The model under review builds one solid part; all positions refer to its coordinate system, in mm. A direction names the side the tool comes from. Round coordinates to 2 decimals unless told otherwise and drop trailing zeros. Loops run counter-clockwise (first coordinate to the right, second up) from the corner with the lowest first, then second, coordinate; pieces in that order, holes last. Notation, with made-up numbers: M 20.25,80 L 55.25,80 A5 ccw 55.25,84 Z; hole C 47.25,56 d11. An arc over 180 degrees is marked long. Return JSON: item names as keys, results as strings. Group by question number.
Q1. Consider section A-A (x = 10). State the section outline as (y, z) points, and give its area (3 significant figures).
Q2. Clearance check with flat-ended pins moving along their axes: pin 1 Ø4.5 at (x, z) = (10, 7.5) entering from +Y; pin 2 Ø0.8 at (y, z) = (0.5, 5.5) entering from -X; pin 3 Ø3 at (x, z) = (14, 3) entering from +Y. State where each tip first meets the part, or that it passes through.
Q3. Consider section C-C (y = 2.5). State the section outline as (x, z) points.
Q4. Draft analysis for pull direction Z (two halves, no side actions). For faces 1 (the face through (32, 0, 8)), 2 (the face through (32.61, 0.45, 0.43)), 3 (the face through (8, 4, 9)), state which applies: pulls with the +Z half, pulls with the -Z half, needs draft (parallel to the pull), parting line crosses it, or undercut.
Q5. Consider section D-D (z = 10.75). State the section outline as (x, y) points, and give its area (3 significant figures).
Q6. For faces 4 (the face through (25, 7, 8)), 5 (the face through (20, 4, 0)), 6 (the face through (25, 1, 8)), list the 3-axis set-ups (+Z, -Z, +X, -X, +Y, -Y) from which the entire face can be reached by the end or side of a thin tool; tool diameter is ignored.
Q7. To check wall thickness, follow line 1 along X through (y, z) = (5.25, 7.5); line 2 along Y through (x, z) = (14, 11.5); line 3 along X through (y, z) = (4, 6). State the ranges of each line that lie inside material, in increasing order.
Q8. Consider section B-B (z = 7.5). State the section outline as (x, y) points.
from build123d import *

# Parameters (mm, degrees)
SKETCH1_W           = 40
SKETCH1_H           = 8
BOSS_EXTRUDE1_DEPTH = 15
SKETCH2_W           = 29.034597986
SKETCH2_H           = 11.917160172
SKETCH2_W_2         = 30.589488345
SKETCH2_H_2         = 7.948253972
CUT_EXTRUDE1_DEPTH  = 15
SKETCH3_R           = 2.5
CUT_EXTRUDE2_DEPTH  = 15
FILLET1_R           = 1.5


with BuildPart() as part:
    # Sketch1 → Boss-Extrude1 (new body)
    with BuildSketch(Plane.XY):
        with Locations((20, 4)):
            Rectangle(SKETCH1_W, SKETCH1_H)
    extrude(amount=BOSS_EXTRUDE1_DEPTH)

    # Sketch2 → Cut-Extrude1 (cut)
    with BuildSketch(Plane.XY.offset(15)):
        with Locations((10.482701007, 12.458580086)):
            Rectangle(SKETCH2_W, SKETCH2_H)
        with Locations((9.705255828, -2.474126986)):
            Rectangle(SKETCH2_W_2, SKETCH2_H_2)
    extrude(amount=-CUT_EXTRUDE1_DEPTH, mode=Mode.SUBTRACT)

    # Sketch3 → Cut-Extrude2 (cut)
    with BuildSketch(Plane(origin=(0, 6.5, 0), x_dir=(1, 0, 0), z_dir=(0, 1, 0))):
        with Locations(Location((10, -7.5, 0), (0, 0, 270))):
            Circle(SKETCH3_R)
    extrude(amount=-CUT_EXTRUDE2_DEPTH, mode=Mode.SUBTRACT)

    # Fillet1
    fillet1_edges = [part.edges().sort_by_distance(p)[0] for p in [
        (32.5, 8, 0),
        (32.5, 0, 0),
    ]]
    fillet(fillet1_edges, radius=FILLET1_R)


solid = part.part
Values:
{
 "1": {"outline": "M 1.5,0 L 6.5,0 L 6.5,5 L 1.5,5 Z; M 1.5,10 L 6.5,10 L 6.5,15 L 1.5,15 Z", "area": "50.0 mm2"},
 "2": {"pin 1": "passes through", "pin 2": "stops at x = 25", "pin 3": "stops at y = 6.5"},
 "3": {"outline": "M 0,0 L 40,0 L 40,15 L 0,15 Z; hole C 10,7.5 d5"},
 "4": {"face 1": "needs draft", "face 2": "pulls with the -Z half", "face 3": "undercut"},
 "5": {"outline": "M 0,1.5 L 25,1.5 L 25,0 L 40,0 L 40,8 L 25,8 L 25,6.5 L 0,6.5 Z", "area": "245 mm2"},
 "6": {"face 4": "+Z, -Z, -X, +Y", "face 5": "-Z, +X, -X, +Y, -Y", "face 6": "+Z, -Z, -X, -Y"},
 "7": {"line 1": "x = 0 to 7.5, 12.5 to 40", "line 2": "y = 1.5 to 6.5", "line 3": "x = 0 to 8, 12 to 40"},
 "8": {"outline": "M 0,1.5 L 7.5,1.5 L 7.5,6.5 L 0,6.5 Z; M 12.5,1.5 L 25,1.5 L 25,0 L 40,0 L 40,8 L 25,8 L 25,6.5 L 12.5,6.5 Z"}
}
